Work out the finished part from the listing and answer in its coordinate system (mm). Face numbers are marked on the shaded views. Give positions to 0.01 mm unless a question says otherwise; leave off trailing zeros. Loops run counter-clockwise (first coordinate to the right, second up) from the corner with the lowest first, then second, coordinate; pieces in that order, holes last. Notation, with made-up numbers: (-29.75, -8.5) -> (9.25, -8.5) arc R19 cw to (9.25, 28.5) -> close; hole circle Ø4 at (30, 32). An arc over 180 degrees is marked (long way). Answer as CSV lines item,"result". Start each with the question number.
1. Find section B-B, the plane z = 1. Give the vertices of the cut face in (x, y), and give its area (3 significant figures).
2. Find section C-C, the plane y = -6.1. Give the vertices of the cut face in (x, z).
3. Find section D-D, the plane x = -4. Give the vertices of the cut face in (y, z), and give its area (3 significant figures).
4. Find section A-A, the plane x = 2. Give the vertices of the cut face in (y, z), and give its area (3 significant figures).
5. Find the intervals of material crossed by line 1 along Y through (x, z) = (2, 0.9); line 2 along Y through (x, z) = (-3.85, 0.6); line 3 along Y through (x, z) = (-2.5, 0.45), in increasing order.
6. Determine the mould class of the marked faces 1 and 2 for opening direction Y: +Y half, -Y half, draft (parallel to the pull), parting line (faces both ways), or undercut.
Autodesk Inventor part; units mm, degrees
ref_plane "YZ Plane" through (0, 0, 0) normal (1, 0, 0) x (0, 1, 0)
ref_plane "XZ Plane" through (0, 0, 0) normal (0, 1, 0) x (-1, 0, 0)
ref_plane "XY Plane" through (0, 0, 0) normal (0, 0, 1) x (1, 0, 0)
sketch "Szkic1" plane through (0, 0, 0) normal (0, 0, 1) x (1, 0, 0)
  line L0 (6.35, -12.7) -> (-6.35, -12.7)
  line L1 (-6.35, -12.7) -> (-6.35, 12.7)
  line L2 (-6.35, 12.7) -> (6.35, 12.7)
  line L3 (6.35, 12.7) -> (6.35, -12.7)
  line L4 (6.35, -12.7) -> (-6.35, 12.7) construction
  line L5 (-6.35, -12.7) -> (6.35, 12.7) construction
  point P0 (0, 0)
  dimension "d0" = 12.7
  dimension "d1" = 25.4
extrude "Wyciągnięcie proste1" add sketch "Szkic1" along normal blind 2
fillet "Zaokrąglenie1" radius 0.5 12 edges at (0, 12.7, 2) (0, 12.7, 0) (-6.35, 12.7, 1) (6.35, 12.7, 1) (6.35, 0, 2) (6.35, 0, 0) (6.35, -12.7, 1) (0, -12.7, 2) (-6.35, 0, 2) (-6.35, -12.7, 1) (-6.35, 0, 0) (0, -12.7, 0)
sketch "Szkic2" plane through (0, 0, 0) normal (0, 0, -1) x (-1, 0, 0)
  line L0 (-5.85, -12.2) -> (5.85, -12.2)
  line L1 (-5.85, -12.2) -> (-5.85, -6.1)
  line L2 (-5.85, 12.2) -> (-5.85, -12.2)
  line L3 (-5.85, -6.1) -> (-3.85, -6.1)
  line L4 (5.85, -12.2) -> (5.85, 12.2)
  line L5 (5.85, -12.2) -> (3.85, -12.2)
  line L6 (3.85, -12.2) -> (3.85, -10.2)
  circle A0 centre (-3.85, -6.1) radius 1.5
  circle A1 centre (3.85, -10.2) radius 1.5
  line L7 (5.85, 12.2) -> (-5.85, 12.2)
  line L8 (-5.85, 12.2) -> (-5.85, 11.2)
  line L9 (0, 12.2) -> (0, 11.2)
  line L10 (0, 11.2) -> (-2, 11.2)
  line L11 (-2, 11.2) -> (-4, 11.2)
  line L12 (0, 11.2) -> (2, 11.2)
  line L13 (2, 11.2) -> (4, 11.2)
  circle A2 centre (-4, 11.2) radius 0.75
  circle A3 centre (-2, 11.2) radius 0.75
  circle A4 centre (0, 11.2) radius 0.75
  circle A5 centre (2, 11.2) radius 0.75
  circle A6 centre (4, 11.2) radius 0.75
  point P0 (0, 0)
  dimension "d5" = 6.1
  dimension "d8" = 2
  dimension "d9" = 2
  dimension "d10" = 2
  dimension "d11" = 3
  dimension "d12" = 3
  dimension "d13" = 1
  dimension "d14" = 1
  dimension "d15" = 2
  dimension "d16" = 2
  dimension "d17" = 2
  dimension "d18" = 2
  dimension "d19" = 1.5
  dimension "d20" = 1.5
  dimension "d21" = 1.5
  dimension "d22" = 1.5
  dimension "d23" = 1.5
extrude "Wyciągnięcie proste2" cut sketch "Szkic2" against normal blind 2 contours A1 | A6 | A5 L13 L12 | L12 L13 A5 | A2 | A3 L11 L10 | L10 L11 A3 | A4 L12 L9 | L9 L10 A4 | A0 | L12 A4 L10
properties part number "Czujnik AltIMU-10"
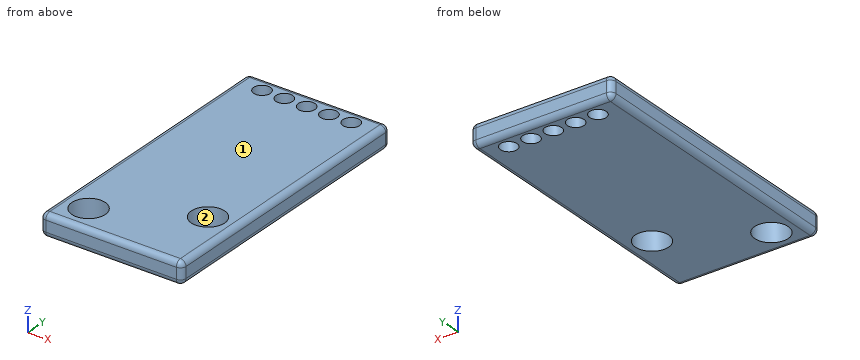
Resolved:
1,outline,"(-6.35, -12.2) arc R0.5 ccw to (-5.85, -12.7) -> (5.85, -12.7) arc R0.5 ccw to (6.35, -12.2) -> (6.35, 12.2) arc R0.5 ccw to (5.85, 12.7) -> (-5.85, 12.7) arc R0.5 ccw to (-6.35, 12.2) -> close; hole circle Ø3 at (-3.85, -10.2); hole circle Ø1.5 at (-4, 11.2); hole circle Ø1.5 at (-2, 11.2); hole circle Ø1.5 at (0, 11.2); hole circle Ø1.5 at (2, 11.2); hole circle Ø3 at (3.85, -6.1); hole circle Ø1.5 at (4, 11.2)"
1,area,"299 mm^2"
2,outline,"(-6.35, 0.5) arc R0.5 ccw to (-5.85, 0) -> (2.35, 0) -> (2.35, 2) -> (-5.85, 2) arc R0.5 ccw to (-6.35, 1.5) -> close; (5.35, 0) -> (5.85, 0) arc R0.5 ccw to (6.35, 0.5) -> (6.35, 1.5) arc R0.5 ccw to (5.85, 2) -> (5.35, 2) -> close"
3,outline,"(-12.7, 0.5) arc R0.5 ccw to (-12.2, 0) -> (-11.69, 0) -> (-11.69, 2) -> (-12.2, 2) arc R0.5 ccw to (-12.7, 1.5) -> close; (-8.71, 0) -> (10.45, 0) -> (10.45, 2) -> (-8.71, 2) -> close; (11.95, 0) -> (12.2, 0) arc R0.5 ccw to (12.7, 0.5) -> (12.7, 1.5) arc R0.5 ccw to (12.2, 2) -> (11.95, 2) -> close"
3,area,"41.6 mm^2"
4,outline,"(-12.7, 0.5) arc R0.5 ccw to (-12.2, 0) -> (10.45, 0) -> (10.45, 2) -> (-12.2, 2) arc R0.5 ccw to (-12.7, 1.5) -> close; (11.95, 0) -> (12.2, 0) arc R0.5 ccw to (12.7, 0.5) -> (12.7, 1.5) arc R0.5 ccw to (12.2, 2) -> (11.95, 2) -> close"
4,area,"47.6 mm^2"
5,line 1,"y = -12.7 to 10.45, 11.95 to 12.7"
5,line 2,"y = -12.7 to -11.7, -8.7 to 10.47, 11.93 to 12.7"
5,line 3,"y = -12.7 to -10.85, -9.55 to 10.64, 11.76 to 12.7"
6,face 1,"draft"
6,face 2,"undercut"
